Part model, mm, in its own coordinate system. Face numbers are marked on the shaded views. A direction names the side the tool comes from. Give positions to 0.01 mm unless a question says otherwise; leave off trailing zeros. Order: outer loops, then holes, each group sorted by start corner. A loop starts at its lowest first (then second) coordinate and runs counter-clockwise, first axis right, second up. Notation, with made-up numbers: M 29,10.25 L 75,10.25 A29 ccw 75,42.25 Z; hole C 84,-10.5 d10. An arc over 180 degrees is marked long. Return JSON: item names as keys, results as strings.
from build123d import *

# Parameters (mm, degrees)
F0_R     = 6.35
F1_DEPTH = 19.05
F2_R     = 20.6375
F3_DEPTH = 25.4


with BuildPart() as f1:
    # F0 (on Top) → F1 (new body)
    with BuildSketch(Plane.XY):
        with BuildLine():
            Line((-50.301953, -7.9375), (-63.001953, -7.9375))
            ThreePointArc((-63.001953, -7.9375), (63.5, 0), (-63.001953, 7.9375))
            Line((-63.001953, 7.9375), (-50.301953, 7.9375))
            Line((-50.301953, 7.9375), (-50.301953, -7.9375))
        make_face()
        with Locations((0, -44.45)):
            Circle(F0_R, mode=Mode.SUBTRACT)
        with Locations((0, 44.45)):
            Circle(F0_R, mode=Mode.SUBTRACT)
        with Locations((44.45, 0)):
            Circle(F0_R, mode=Mode.SUBTRACT)
    extrude(amount=F1_DEPTH)

    # F2 (on face) → F3 (join)
    with BuildSketch(Plane.XY.offset(19.05)):
        Circle(F2_R)
    extrude(amount=F3_DEPTH)


solid = f1.part
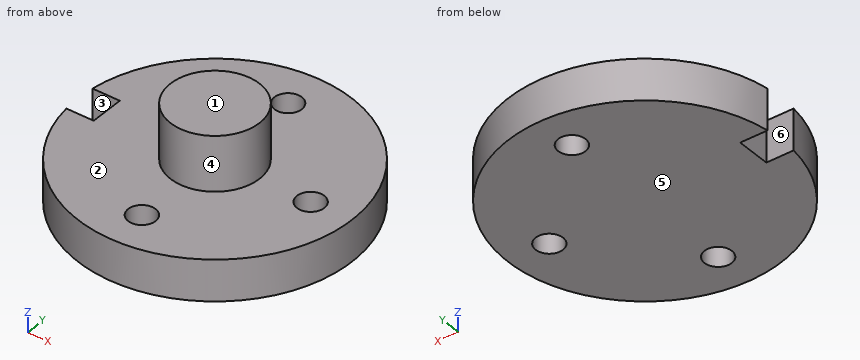
Q1. Probe line 1 along Y through (x, z) = (0, 15.25); line 2 along Z through (x, y) = (-23, -7); line 3 along X through (y, z) = (-42.5, 9.5). List the from-to ranges inside material, lowest first.
Established:
{"line 1": "y = -63.5 to -50.8, -38.1 to 38.1, 50.8 to 63.5", "line 2": "z = 0 to 19.05", "line 3": "x = -47.18 to -6.04, 6.04 to 47.18"}
Q2. Band-saw the part on A-A (x = 0). Give the cut face in (y, z), then the cut area to 3 significant figures.
Established:
{"outline": "M -63.5,0 L -50.8,0 L -50.8,19.05 L -63.5,19.05 Z; M -38.1,0 L 38.1,0 L 38.1,19.05 L 20.64,19.05 L 20.64,44.45 L -20.64,44.45 L -20.64,19.05 L -38.1,19.05 Z; M 50.8,0 L 63.5,0 L 63.5,19.05 L 50.8,19.05 Z", "area": "2,980 mm²"}
Q3. Band-saw the part on B-B (z = 12.5). Give the cut face in (x, y).
Established:
{"outline": "M -63,-7.94 A63.5 ccw long -63,7.94 L -50.3,7.94 L -50.3,-7.94 Z; hole C 0,-44.45 d12.7; hole C 0,44.45 d12.7; hole C 44.45,0 d12.7"}
Q4. 3-axis set-ups, long thin cutter, end or side, ignore diameter. For the marked faces 1, 2 and 3: which of +Z, -Z, +X, -X, +Y, -Y reach the whole face in a straight line?
Established:
{"face 1": "+Z, +X, -X, +Y, -Y", "face 2": "+Z", "face 3": "+Z, -Z, -X"}
Q5. Pin check, flat tips, straight feed: pin 1 (3 mm diameter, centred on y = -1, z = 32.5, fed in from +X); pin 2 (12 mm diameter, centred on y = 16, z = 22, fed in from +X); pin 3 (6 mm diameter, centred on x = 24.5, z = 5, fed in from -Y). Stop position of each tip, or through.
Established:
{"pin 1": "stops at x = 20.64", "pin 2": "stops at x = 62.58", "pin 3": "stops at y = -59.75"}
Q6. Band-saw the part on C-C (y = 44.45). Give the cut face in (x, z).
Established:
{"outline": "M -45.35,0 L -6.35,0 L -6.35,19.05 L -45.35,19.05 Z; M 6.35,0 L 45.35,0 L 45.35,19.05 L 6.35,19.05 Z"}
Q7. Two-plate mould, pull along Y, no slides. Class the marked faces 4, 5 and 6: +Y half, -Y half, draft (parallel to the pull), parting line (faces both ways), or undercut.
Established:
{"face 4": "parting line", "face 5": "draft", "face 6": "undercut"}
